Build history of the part. All positions in model axes, mm. Face numbers are marked on the shaded views. Round coordinates to 2 decimals unless told otherwise and drop trailing zeros. Write each loop counter-clockwise with the first axis right and the second up, starting at its lowest first coordinate (ties: lowest second). Pieces come first, ordered by that corner, then holes. Notation, with made-up numbers: (3.25, 47.25) - (43.25, 47.25) arc R21 cw to (43.25, 86.25) - close; hole circle Ø11 at (-22.5, -22.5). An arc over 180 degrees is marked (long way). One line per question, with ' | ' between items.
from build123d import *

# Parameters (mm, degrees)
F0_W        = 2.54
F0_H        = 3.81
F0_W_2      = 3.81
F0_H_2      = 73.66
F1_DEPTH    = 3.175
F2_DEPTH    = 9.7028
F3_START    = 6.35
F3_DEPTH    = 3.3528
F5_DEPTH    = 2.54
F6_T2_ANGLE = 26.9228721227
F6_T4_ANGLE = 124.2205290786
F6_T6_ANGLE = 26.9228721227


# Not quite as in the source:
# - a fillet or chamfer that OpenCascade refuses, or shapes differently, is made with other operations: its cross-section is extruded or revolved along the edge and cut away or added


with BuildPart() as f1:
    # F0 (on Top) → F1 (new body)
    with BuildSketch(Plane.XY):
        Polygon((-55.88, -36.83), (-55.88, 36.83), (55.88, 36.83), (59.69, 36.83), (59.69, 40.64), (-59.69, 40.64), (-59.69, -40.64), (59.69, -40.64), (59.69, -36.83), (55.88, -36.83), align=None)
        with Locations((60.96, 38.735)):
            Rectangle(F0_W, F0_H)
        with Locations((60.96, -38.735)):
            Rectangle(F0_W, F0_H)
        with Locations((57.785, 0)):
            Rectangle(F0_W_2, F0_H_2)
        with Locations((60.96, 0)):
            Rectangle(F0_W, F0_H_2)
    extrude(amount=F1_DEPTH)

    # F0 (on Top) → F2 (join)
    with BuildSketch(Plane.XY):
        Polygon((-59.69, 40.64), (59.69, 40.64), (62.23, 40.64), (62.23, 43.18), (-62.23, 43.18), (-62.23, -43.18), (62.23, -43.18), (62.23, -40.64), (59.69, -40.64), (-59.69, -40.64), align=None)
    extrude(amount=F2_DEPTH)

    # F0 (on Top) → F3 (join)
    with BuildSketch(Plane.XY.offset(F3_START)):
        Polygon((-55.88, -36.83), (-55.88, 36.83), (55.88, 36.83), (59.69, 36.83), (59.69, 40.64), (-59.69, 40.64), (-59.69, -40.64), (59.69, -40.64), (59.69, -36.83), (55.88, -36.83), align=None)
        with Locations((60.96, -38.735)):
            Rectangle(F0_W, F0_H)
        with Locations((60.96, 38.735)):
            Rectangle(F0_W, F0_H)
    extrude(amount=F3_DEPTH)

    # F4 (on face) → F5 (join)
    with BuildSketch(Plane(origin=(0, 0, 0), x_dir=(1, 0, 0), z_dir=(0, 0, -1))):
        with BuildLine():
            Line((33.6746639179, 36.83), (-33.6746639179, 36.83))
            ThreePointArc((-33.6746639179, 36.83), (0, 16.5520933119), (33.6746639179, 36.83))
        make_face()
        with BuildLine():
            Line((36.331819044, 43.18), (-36.331819044, 43.18))
            ThreePointArc((-36.331819044, 43.18), (-35.1469421027, 39.9448685285), (-33.6746639179, 36.83))
            Line((-33.6746639179, 36.83), (33.6746639179, 36.83))
            ThreePointArc((33.6746639179, 36.83), (35.1469421027, 39.9448685285), (36.331819044, 43.18))
        make_face()
    extrude(amount=F5_DEPTH)

    # F6: fillet of radius 5.08 on 1 edges, made by hand

    # F6_s1 → F6_t2 (revolve, cut)
    with BuildSketch(Plane(origin=(-0.9220761964, -54.6365318462, 0), x_dir=(0, 0, 1), z_dir=(-0.0168741478, -0.9998576214, 0))):
        with BuildLine():
            ThreePointArc((0, 37.177792501), (-1.8594090512, 35.3183834498), (-2.54, 32.7783834498))
            Line((-2.54, 32.7783834498), (-2.54, 37.177792501))
            Line((-2.54, 37.177792501), (0, 37.177792501))
        make_face()
    revolve(axis=Axis((0, -54.6520933119, -2.54), (0, 0, -1)), revolution_arc=F6_T2_ANGLE, mode=Mode.SUBTRACT)

    # F6_s3 → F6_t4 (revolve, cut)
    with BuildSketch(Plane(origin=(-22.5953375952, -42.6936601597, 0), x_dir=(0, 0, 1), z_dir=(-0.4677714801, -0.8838494455, 0))):
        with BuildLine():
            ThreePointArc((0, 12.5353094191), (-1.8594090512, 10.6759003679), (-2.54, 8.1359003679))
            Line((-2.54, 8.1359003679), (-2.54, 12.5353094191))
            Line((-2.54, 12.5353094191), (0, 12.5353094191))
        make_face()
    revolve(axis=Axis((0, -54.6520933119, -2.54), (0, 0, -1)), revolution_arc=F6_T4_ANGLE, mode=Mode.SUBTRACT)

    # F6_s5 → F6_t6 (revolve, cut)
    with BuildSketch(Plane(origin=(22.5953375952, -42.6936601597, 0), x_dir=(0, 0, 1), z_dir=(-0.4677714801, 0.8838494455, 0))):
        with BuildLine():
            ThreePointArc((0, 12.5353094191), (-1.8594090512, 10.6759003679), (-2.54, 8.1359003679))
            Line((-2.54, 8.1359003679), (-2.54, 12.5353094191))
            Line((-2.54, 12.5353094191), (0, 12.5353094191))
        make_face()
    revolve(axis=Axis((0, -54.6520933119, -2.54), (0, 0, -1)), revolution_arc=F6_T6_ANGLE, mode=Mode.SUBTRACT)


solid = f1.part
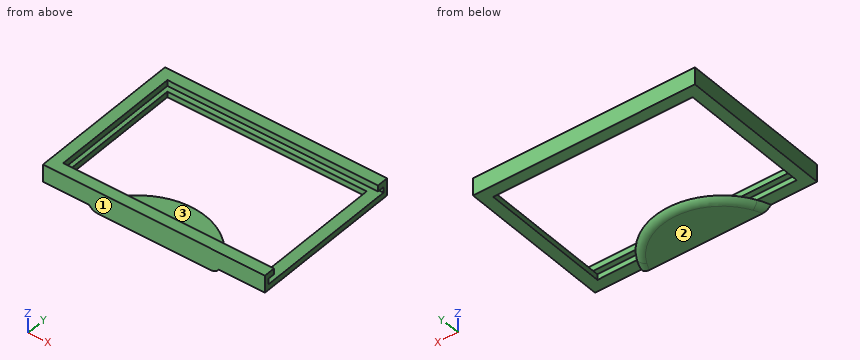
Q1. Saw through at B-B, the plane z = 1.5. List the corners of the cut face in (x, y).
Found:
outline: (-62.23, -43.18) - (62.23, -43.18) - (62.23, 43.18) - (-62.23, 43.18) - close; hole (-55.88, -36.83) - (55.88, -36.83) - (55.88, 36.83) - (-55.88, 36.83) - close
Q2. Saw through at A-A, the plane x = 45.5. List the corners of the cut face in (y, z) (3 decimals), then the cut area to 3 significant figures.
Found:
outline: (-43.18, 0) - (-36.83, 0) - (-36.83, 3.175) - (-40.64, 3.175) - (-40.64, 6.35) - (-36.83, 6.35) - (-36.83, 9.703) - (-43.18, 9.703) - close; (36.83, 0) - (43.18, 0) - (43.18, 9.703) - (36.83, 9.703) - (36.83, 6.35) - (40.64, 6.35) - (40.64, 3.175) - (36.83, 3.175) - close | area: 99.0 mm^2
Q3. Drop flat-ended pins along their axis: pin 1 (1 mm diameter, centred on y = 1.5, z = 4.5, fed in from +X); pin 2 (2.5 mm diameter, centred on y = -0.5, z = 8, fed in from +X); pin 3 (24.5 mm diameter, centred on x = -4, y = 13.5, fed in from -Z); pin 4 (10 mm diameter, centred on x = -11, y = -25, fed in from +Z). Give the stop position or say it passes through.
Found:
pin 1: x = -59.69 | pin 2: x = -55.88 | pin 3: through | pin 4: z = 0
Q4. Drill centre lines: L1, parallel to Z at x = 56, y = 37.5 (3 decimals); L2, parallel to Y at x = 19, z = 7; L3, parallel to X at y = -31.5, z = 0.25. Where is each one in solid material? Low to high. Write a range as from..to.
Found:
L1: 0..3.175, 6.35..9.703 | L2: -43.18..-36.83, 36.83..43.18 | L3: -62.23..-55.88, 55.88..62.23
Q5. Saw through at C-C, the plane y = 15.5. List the corners of the cut face in (x, z) (3 decimals), then the cut area to 3 significant figures.
Found:
outline: (-62.23, 0) - (-55.88, 0) - (-55.88, 3.175) - (-59.69, 3.175) - (-59.69, 6.35) - (-55.88, 6.35) - (-55.88, 9.703) - (-62.23, 9.703) - close; (55.88, 0) - (62.23, 0) - (62.23, 3.175) - (55.88, 3.175) - close | area: 69.7 mm^2
Q6. Pull direction Y, two halves, no side cores. Call the marked faces 1, 2 and 3: +Y half, -Y half, draft (parallel to the pull), parting line (faces both ways), or undercut.
Found:
face 1: -Y half | face 2: draft | face 3: undercut
Q7. Saw through at D-D, the plane y = -18. State how many separate pieces and enclosed holes the cut face has, then the cut area to 3 significant figures.
Found:
separate pieces: 3 | enclosed holes: 0 | area: 93.6 mm^2
